```python
from build123d import *

# Parameters (mm, degrees)
BOSS_EXTRU_2_DEPTH      = 2
CONG_1_R                = 1
ESQUISSE2_R             = 1
ESQUISSE2_R_2           = 1.5
ENL_V_MAT_EXTRU_1_DEPTH = 50.654670275
CONG_2_R                = 2.5


with BuildPart() as part:
    # Esquisse1 → Boss.-Extru.2 (new body)
    with BuildSketch(Plane.XY):
        with BuildLine():
            Line((0.95447274, 5.745584386), (3.449873287, -1.110472271))
            Line((3.449873287, -1.110472271), (8.449873287, -1.110472271))
            Line((8.449873287, -1.110472271), (7.995996013, 0.174830759))
            ThreePointArc((7.995996013, 0.174830759), (5.44417176, 1.394745914), (6.664086914, 3.946570166))
            Line((6.664086914, 3.946570166), (6.564193732, 4.229450622))
            ThreePointArc((6.564193732, 4.229450622), (4.012369479, 5.449365776), (5.232284634, 8.001190029))
            Line((5.232284634, 8.001190029), (5.132391451, 8.284070484))
            ThreePointArc((5.132391451, 8.284070484), (2.580567198, 9.503985638), (3.800482353, 12.055809891))
            Line((3.800482353, 12.055809891), (3.70058917, 12.338690347))
            ThreePointArc((3.70058917, 12.338690347), (1.148764918, 13.558605501), (2.368680072, 16.110429753))
            Line((2.368680072, 16.110429753), (2.360851147, 16.132599934))
            ThreePointArc((2.360851147, 16.132599934), (4.854316205, 19.307619995), (3.042318195, 22.915220804))
            ThreePointArc((3.042318195, 22.915220804), (1.102078927, 25.284293174), (3.769763015, 26.787787077))
            Line((3.769763015, 26.787787077), (3.87507245, 27.068696178))
            ThreePointArc((3.87507245, 27.068696178), (2.663964414, 29.524327439), (5.038572788, 30.887464495))
            ThreePointArc((5.038572788, 30.887464495), (7.001105436, 32.201717881), (5.901338085, 34.292006887))
            ThreePointArc((5.901338085, 34.292006887), (3.997941168, 36.347217372), (6.01632714, 38.289620015))
            Line((6.01632714, 38.289620015), (6.019210973, 38.589804586))
            ThreePointArc((6.019210973, 38.589804586), (4.038516109, 40.608925151), (6.057636674, 42.589620015))
            Line((6.057636674, 42.589620015), (6.060520508, 42.889804586))
            ThreePointArc((6.060520508, 42.889804586), (4.079825644, 44.908925151), (6.098946209, 46.889620015))
            Line((6.098946209, 46.889620015), (6.11815906, 48.889527729))
            Line((6.11815906, 48.889527729), (2.631980822, 46.876781785))
            Line((2.631980822, 46.876781785), (-5.50821759, 24.511770458))
            Line((-5.50821759, 24.511770458), (-5.50821759, 12.511770458))
            Line((-5.50821759, 12.511770458), (-3.04552726, 5.745584386))
            Line((-3.04552726, 5.745584386), (0.95447274, 5.745584386))
        make_face()
    extrude(amount=BOSS_EXTRU_2_DEPTH)

    # Congé1
    cong_1_edges = [part.edges().sort_by_distance(p)[0] for p in [
        (6.098946209, 46.889620015, 1),
    ]]
    fillet(cong_1_edges, radius=CONG_1_R)

    # Esquisse2 → Enlèv. mat.-Extru.1 (cut, through all)
    with BuildSketch(Plane.XY.offset(2)):
        with Locations((2.016979912, 38.376781785)):
            Circle(ESQUISSE2_R)
        with Locations((1.092901094, 33.876781785)):
            Circle(ESQUISSE2_R_2)
        with Locations((-1.50821759, 19.511770458)):
            Circle(ESQUISSE2_R_2)
        with Locations((-1.50821759, 24.511770458)):
            Circle(ESQUISSE2_R)
    extrude(amount=-ENL_V_MAT_EXTRU_1_DEPTH, mode=Mode.SUBTRACT)

    # Congé2
    # the kernel refuses this fillet: 2.5 mm, written as the material it adds along each edge
    with BuildSketch(Plane(origin=(0.95447274, 5.745584386, 0), x_dir=(-1, 0, 0), z_dir=(0, 0, 1))) as cong_2_piece_1:
        with BuildLine():
            CenterArc((CONG_2_R * 0.70020753821, CONG_2_R), CONG_2_R, 200, 70)
            Line((-CONG_2_R * 0.239485082576, CONG_2_R * 0.657979856674), (0, 0))
            Line((0, 0), (CONG_2_R * 0.70020753821, 0))
        make_face()
    extrude(amount=2)
    # the kernel refuses this fillet: 2.5 mm, written as the material it takes off along each edge
    with BuildSketch(Plane(origin=(8.449873287, -1.110472271, -6.597356953), x_dir=(-1, 0, 0), z_dir=(0, 0, 1))) as cong_2_2_piece_1:
        with BuildLine():
            CenterArc((2.638942781, -2.5), CONG_2_R, 90, 60.929935742)
            Line((0.453877274, -1.28530303), (0, 0))
            Line((0, 0), (2.638942781, 0))
        make_face()
    extrude(amount=15.194713907, mode=Mode.SUBTRACT)
    with BuildSketch(Plane(origin=(3.449873287, -1.110472271, -4.376297114), x_dir=(-0.3420201433256723, 0.9396926207859071, 0), z_dir=(0, 0, 1)), Plane(origin=(-3.04552726, 5.745584386, -4.376297114), x_dir=(-0.34202014332566605, 0.9396926207859094, 0), z_dir=(0, 0, 1))) as cong_2_2_piece_2:
        with BuildLine():
            CenterArc((CONG_2_R * 0.70020753821, -CONG_2_R), CONG_2_R, 90, 70)
            Line((-CONG_2_R * 0.239485082576, -CONG_2_R * 0.657979856674), (0, 0))
            Line((0, 0), (CONG_2_R * 0.70020753821, 0))
        make_face()
    extrude(amount=10.752594228, mode=Mode.SUBTRACT)


solid = part.part
```
Source: CAD feature listing. Evaluate the final solid. Frame: model axes, mm. A direction names the side the tool comes from. Give positions to 0.01 mm unless a question says otherwise; leave off trailing zeros. Order: outer loops, then holes, each group sorted by start corner. A loop starts at its lowest first (then second) coordinate and runs counter-clockwise, first axis right, second up.
(1) Pull-direction query (Y, two-part tool) for faces 3 (the face through (3.997, 36.304, 0.986)), 4 (the face through (-4.59, 9.99, 0.99)), 5 (the face through (0, 24, 0)); classes: +Y half, -Y half, draft (parallel to the pull), parting line (faces both ways), or undercut.
(2) Contact query for flat-ended pins moving along their axis: P1, Ø1, axis at x = 4.5, z = 1.5, coming from the -Y side; P2, Ø0.5, axis at x = -1, z = 0.5, coming from the -Y side; P3, Ø1.6, axis at x = 2.02, y = 38.38, coming from the +Z side. Output: stop coordinate, or through.
(3) Section query C-C (z = 1.1). State how many separate pieces and enclosed holes the cut face has, plus the area to 3 significant figures.
(4) Section query A-A (x = -1.75). Return the cut outline in (y, z), plus the area to 3 significant figures.
(5) Access query for faces 1 (the face through (0, 24, 2)), 2 (the face through (5.913, 47.135, 1.014)). Directions: +Z, -Z, +X, -X, +Y, -Y. A direction counts if a zero-diameter tool reaches every point of the face in a straight line with its end or side. Return the directions, or none.
(6) Material intervals for line 1 along X through (y, z) = (22, 1.85); line 2 along X through (y, z) = (6, 0.85), sorted ascending.
(7) Section query B-B (y = 9). Return the cut outline in (x, z), plus the area to 3 significant figures.
(8) Section query D-D (y = 45.5). Return the cut outline in (x, z).
Outcome:
1. face 3: undercut
1. face 4: -Y half
1. face 5: draft
2. P1: stops at y = -1.1
2. P2: stops at y = 5.75
2. P3: passes through
3. separate pieces: 1
3. enclosed holes: 4
3. area: 288 mm2
4. outline: (5.79, 0) - (18.03, 0) - (18.03, 2) - (5.79, 2) - close; (20.99, 0) - (23.54, 0) - (23.54, 2) - (20.99, 2) - close; (25.48, 0) - (34.84, 0) - (34.84, 2) - (25.48, 2) - close
4. area: 48.3 mm2
5. face 1: +Z, +X, -X, +Y, -Y
5. face 2: +Z, -Z, +X
6. line 1: x = -5.51 to 4.08
6. line 2: x = -2.39 to 3.9
7. outline: (-4.23, 0) - (2.84, 0) - (2.84, 2) - (-4.23, 2) - close
7. area: 14.1 mm2
8. outline: (2.13, 0) - (4.18, 0) - (4.18, 2) - (2.13, 2) - close
